Source: three-view drawing plus pictorial views. Frame: mm from the lowest corner of the part. A direction names the side the tool comes from. Give positions to 0.01 mm unless a question says otherwise; leave off trailing zeros. Order: outer loops, then holes, each group sorted by start corner. A loop starts at its lowest first (then second) coordinate and runs counter-clockwise, first axis right, second up. Notation, with made-up numbers: (40.25, 58.5) - (61.25, 58.5) arc R28 cw to (61.25, 92.5) - close; hole circle Ø5 at (19.5, 69). An arc over 180 degrees is marked (long way). Use one line per item in the form item = value.
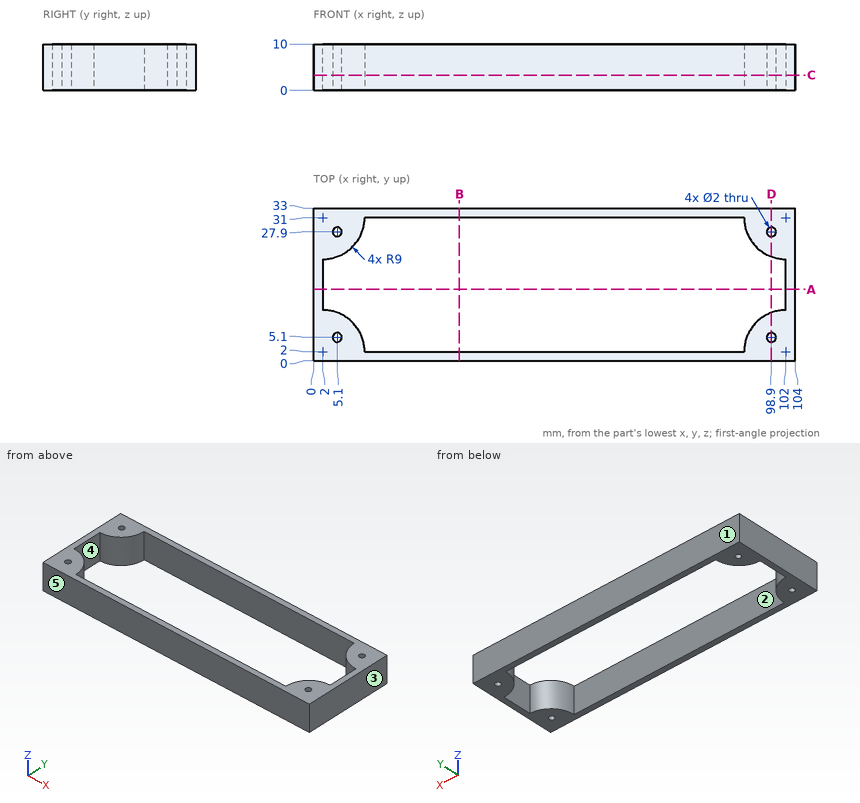
(1) Cut plane C-C on z = 3.25. Output: boundary loops of the cut face in (x, y), plus the area to 3 significant figures.
Computed values:
outline = (0, 0) - (104, 0) - (104, 33) - (0, 33) - close; hole (2, 11) arc R9 cw to (11, 2) - (93, 2) arc R9 cw to (102, 11) - (102, 22) arc R9 cw to (93, 31) - (11, 31) arc R9 cw to (2, 22) - close; hole circle Ø2 at (5.1, 5.1); hole circle Ø2 at (5.1, 27.9); hole circle Ø2 at (98.9, 5.1); hole circle Ø2 at (98.9, 27.9)
area = 774 mm²
(2) Ray query, line 1 along Y through (x, z) = (17, 9.75); line 2 along Y through (x, z) = (98.9, 5); line 3 along X through (y, z) = (15, 4.5). Return the intervals inside material, ascending.
Computed values:
line_1 = 0 to 2, 31 to 33
line_2 = 0 to 4.1, 6.1 to 10.45, 22.55 to 26.9, 28.9 to 33
line_3 = 0 to 2, 102 to 104
(3) Cut plane B-B on x = 31.5. Output: boundary loops of the cut face in (y, z).
Computed values:
outline = (0, 0) - (2, 0) - (2, 10) - (0, 10) - close; (31, 0) - (33, 0) - (33, 10) - (31, 10) - close
(4) Cut plane A-A on y = 15.5. Output: boundary loops of the cut face in (x, z).
Computed values:
outline = (0, 0) - (2, 0) - (2, 10) - (0, 10) - close; (102, 0) - (104, 0) - (104, 10) - (102, 10) - close
(5) Reachability of the marked faces 4 and 5 from +Z, -Z, +X, -X, +Y, -Y: full face, straight path, thin tool, end or side. Return the list, or none.
Computed values:
face_4 = +Z, -Z
face_5 = +Z, -Z, +X, -X, -Y
(6) Contact query for a flat-ended pin moving along its axis: pin 1 Ø1.6 at (x, y) = (5.1, 27.9) entering from -Z. Output: stop coordinate, or through.
Computed values:
pin_1 = through
(7) Cut plane D-D on x = 98.9. Output: boundary loops of the cut face in (y, z).
Computed values:
outline = (0, 0) - (4.1, 0) - (4.1, 10) - (0, 10) - close; (6.1, 0) - (10.45, 0) - (10.45, 10) - (6.1, 10) - close; (22.55, 0) - (26.9, 0) - (26.9, 10) - (22.55, 10) - close; (28.9, 0) - (33, 0) - (33, 10) - (28.9, 10) - close
(8) Pull-direction query (X, two-part tool) for the marked faces 1, 2 and 3; classes: released by +X, released by -X, zero draft, split by the parting line, or undercut.
Computed values:
face_1 = zero draft
face_2 = undercut
face_3 = released by +X
